Part model, mm, in its own coordinate system. A direction names the side the tool comes from. Round coordinates to 2 decimals unless told otherwise and drop trailing zeros. Loops run counter-clockwise (first coordinate to the right, second up) from the corner with the lowest first, then second, coordinate; pieces in that order, holes last.
Autodesk Inventor part; units mm, degrees
ref_plane "YZ Plane" through (0, 0, 0) normal (1, 0, 0) x (0, 1, 0)
ref_plane "XZ Plane" through (0, 0, 0) normal (0, 1, 0) x (-1, 0, 0)
ref_plane "XY Plane" through (0, 0, 0) normal (0, 0, 1) x (1, 0, 0)
sketch "Sketch3" plane through (0, 0, 0) normal (0, 1, 0) x (-1, 0, 0)
  line L0 (0, 0) -> (-55, 0)
  line L1 (-55, 0) -> (-55, -35.25)
  line L2 (-55, -35.25) -> (0, -35.25)
  line L3 (0, -35.25) -> (0, 0)
  line L4 (1.5, 1.5) -> (-56.5, 1.5)
  line L5 (-56.5, 1.5) -> (-56.5, -36.75)
  line L6 (-56.5, -36.75) -> (1.5, -36.75)
  line L7 (1.5, -36.75) -> (1.5, 1.5)
  dimension "d0" = 35.25
  dimension "d1" = 55
  dimension "d4" = 38.25
  dimension "d5" = 58
  dimension "d6" = 1.5
  dimension "d7" = 1.5
extrude "Extrusion1" add sketch "Sketch3" against normal blind 1.5 contours L3 L2 L1 L0 | L7 L6 L5 L4
sketch "Sketch5" plane through (0, 0, 0) normal (0, 1, 0) x (-1, 0, 0)
  line L0 (-55, 0) -> (-55, -35.25)
  line L1 (-55, -35.25) -> (0, -35.25)
  line L2 (0, -35.25) -> (0, 0)
  line L3 (-56.5, 1.5) -> (-56.5, -36.75)
  line L4 (-56.5, -36.75) -> (1.5, -36.75)
  line L5 (1.5, -36.75) -> (1.5, 1.5)
  line L6 (0, 0) -> (0, 1.5)
  line L7 (1.5, 1.5) -> (0, 1.5)
  line L8 (-55, 0) -> (-55, 1.5)
  line L9 (-55, 1.5) -> (-56.5, 1.5)
  dimension "d9" = 55
  dimension "d11" = 58
  dimension "d12" = 1.5
extrude "Extrusion2" add sketch "Sketch5" along normal blind 28
sketch "Sketch6" plane through (0, 28, 0) normal (0, 1, 0) x (1, 0, 0)
  line L0 (-1.5, -1.5) -> (56.5, -1.5)
  line L1 (56.5, -1.5) -> (56.5, 36.75)
  line L2 (56.5, 36.75) -> (-1.5, 36.75)
  line L3 (-1.5, 36.75) -> (-1.5, -1.5)
  point P0 (0, 0)
extrude "Extrusion3" add sketch "Sketch6" along normal blind 1.5
sketch "Sketch7" plane through (0, 0, 1.5) normal (1, 0, 0) x (0, 0, -1)
  line L0 (8.375, 4.5) -> (23.375, 4.5)
  line L1 (23.375, 4.5) -> (23.375, 5.5)
  line L2 (23.375, 5.5) -> (8.375, 5.5)
  line L3 (8.375, 5.5) -> (8.375, 4.5)
  line L4 (36.75, 0) -> (36.75, 28)
  line L5 (0, 0) -> (0, 28)
  line L6 (36.75, 0) -> (0, 0)
  point P0 (1.5, 0)
  dimension "d20" = 15
  dimension "d21" = 1
  dimension "d22" = 13.375
  dimension "d23" = 8.375
  dimension "d40" = 4.5
ref_plane "Work Plane1" through (27.5, 0, 1.5) normal (1, 0, 0) x (0, 0, -1)
extrude "Extrusion4" add sketch "Sketch7" along normal blind 2
mirror "Mirror1" about plane through (27.5, 0, 1.5) normal (1, 0, 0) of "Extrusion4"
sketch "Sketch8" plane through (-1.5, -1.5, 1.5) normal (0, 0, 1) x (1, 0, 0)
  line L0 (0.75, 30.25) -> (57.25, 30.25)
  line L1 (57.25, 30.25) -> (57.25, 13.25)
  line L2 (0.75, 13.25) -> (0.75, 30.25)
  line L3 (0, 31) -> (58, 31)
  line L4 (0.75, 13.25) -> (0, 13.25)
  line L5 (57.25, 13.25) -> (58, 13.25)
  line L6 (0, 31) -> (0, 13.25)
  line L7 (0, 31) -> (0, 0)
  line L8 (58, 31) -> (58, 13.25)
  line L9 (58, 0) -> (58, 31)
  point P0 (1.5, 1.5)
  dimension "d27" = 0.75
  dimension "d29" = 56.5
  dimension "d31" = 17
  dimension "d65" = 0.75
  dimension "d84" = 17
extrude "Extrusion5" add sketch "Sketch8" along normal blind 3
sketch "Sketch9" plane through (-1.5, -1.5, 1.5) normal (0, 0, 1) x (1, 0, 0)
  line L0 (0.75, 0.75) -> (57.25, 0.75)
  line L1 (57.25, 0.75) -> (57.25, 17.5)
  line L2 (0.75, 17.5) -> (0.75, 0.75)
  line L3 (1.5, 1.5) -> (56.5, 1.5)
  line L4 (57.25, 17.5) -> (56.5, 17.5)
  line L5 (56.5, 1.5) -> (56.5, 29.5)
  line L6 (56.5, 1.5) -> (56.5, 17.5)
  line L7 (56.5, 1.5) -> (1.5, 1.5)
  line L8 (0.75, 17.5) -> (1.5, 17.5)
  line L9 (1.5, 1.5) -> (1.5, 29.5)
  line L10 (1.5, 17.5) -> (1.5, 1.5)
  line L11 (1.5, 29.5) -> (56.5, 29.5)
  dimension "d34" = 0.75
  dimension "d36" = 56.5
  dimension "d69" = 16.75
  dimension "d70" = 16.75
  dimension "d97" = 28.75
extrude "Extrusion6" add sketch "Sketch9" along normal blind 3 contours L2 L8 L9 L3 L5 L4 L1 L0
sketch "Sketch10" plane through (0, 0, -35.25) normal (0, 0, 1) x (1, 0, 0)
  line L0 (55, 0) -> (0, 0)
  line L1 (20.5, 0) -> (34.5, 0)
  line L2 (34.5, 0) -> (34.5, 3.3)
  line L3 (34.5, 3.3) -> (20.5, 3.3)
  line L4 (20.5, 3.3) -> (20.5, 0)
  line L5 (0, 0) -> (0, 28)
  dimension "d41" = 14
  dimension "d42" = 20.5
  dimension "d43" = 3.3
extrude "Extrusion7" add sketch "Sketch10" along normal blind 5
fillet "Fillet1" radius 1 8 edges at (56.5, 29.5, -16.125) (56.5, -1.5, -17.625) (56.5, 14, -36.75) (27.5, 29.5, -36.75) (27.5, -1.5, -36.75) (-1.5, 14, -36.75) (-1.5, 29.5, -16.125) (-1.5, -1.5, -17.625)
sketch "Sketch11" plane through (0, 28, -35.25) normal (0, 0, 1) x (1, 0, 0)
  circle A0 centre (27.5, -17.2) radius 4.95
  line L0 (20.5, -24.7) -> (34.5, -24.7)
  line L1 (0, -28) -> (0, 0)
  dimension "d47" = 9.9
  dimension "d48" = 7.5
  dimension "d49" = 27.5
extrude "Extrusion8" cut sketch "Sketch11" against normal blind 5
fillet "Fillet2" radius 1 1 edges at (-0.75, -0.75, 3)
fillet "Fillet3" radius 1 1 edges at (55.75, -0.75, 3)
sketch "Sketch15" plane through (56.5, 11.75, 4.5) normal (1, 0, 0) x (0, 0, -1)
  line L0 (0, 0) -> (5, 0)
  line L1 (5, 0) -> (5, 12.75)
  line L2 (5, 12.75) -> (0, 12.75)
  line L3 (0, 12.75) -> (0, 0)
  line L4 (5, 0) -> (3, 0)
  line L5 (3, 0) -> (3, -7.25)
  line L6 (3, -7.25) -> (5, -7.25)
  line L7 (5, -7.25) -> (5, 0)
  point P0 (4.5, -11.75)
  point P1 (0, 4.25)
  point P2 (0, 17.75)
  dimension "d78" = 5
  dimension "d79" = 12.75
  dimension "d80" = 2
  dimension "d81" = 7.25
  dimension "d98" = 11.5
  dimension "d99" = 20
  dimension "d100" = 12.75
  dimension "d101" = 5
extrude "Extrusion10" add sketch "Sketch15" along normal blind 5
mirror "Mirror3" about plane through (27.5, 0, 1.5) normal (1, 0, 0) of "Extrusion10"
fillet "Fillet7" radius 1 2 edges at (61.5, 24.5, 2) (61.5, 4.5, 0.5)
fillet "Fillet8" radius 1 2 edges at (-6.5, 24.5, 2) (-6.5, 4.5, 0.5)
sketch "Sketch16" plane through (-1.5, -1.5, 4.5) normal (0, 0, 1) x (1, 0, 0)
  circle A0 centre (60.5, 22.5) radius 1.5
  line L0 (63, 25) -> (63, 13.25)
  line L1 (58, 26) -> (62, 26)
  point P0 (1.5, 1.5)
  dimension "d87" = 3
  dimension "d88" = 2.5
  dimension "d89" = 3.5
extrude "Extrusion11" cut sketch "Sketch16" against normal blind 5
sketch "Sketch17" plane through (-0.5, -1.5, 1.5) normal (0, 0, 1) x (1, 0, 0)
  circle A0 centre (59.5, 9.5) radius 1.5
  line L0 (57, 6) -> (61, 6)
  line L1 (62, 7) -> (62, 25)
  point P0 (0.5, 1.5)
  dimension "d92" = 3
  dimension "d93" = 3.5
  dimension "d94" = 2.5
extrude "Extrusion12" cut sketch "Sketch17" against normal blind 2
mirror "Mirror4" about plane through (27.5, 0, 1.5) normal (1, 0, 0) of "Extrusion11", "Extrusion12"
equation "\"d7\" = d6"
equation "\"d31\" = d66"
equation "\"d70\" = d69"
properties part number "sensor1_2t"
1) Drop flat-ended pins along their axis: pin 1 Ø1 at (y, z) = (7, -30) entering from -X; pin 2 Ø3 at (x, z) = (57.5, 2.5) entering from +Y; pin 3 Ø0.9 at (x, z) = (15.5, 3) entering from -Y; pin 4 Ø6 at (x, y) = (27.5, 10.8) entering from +Z. Give the stop position or say it passes through.
Values:
pin 1: stops at x = -1.5
pin 2: stops at y = 29.37
pin 3: stops at y = -0.75
pin 4: passes through
2) Tool access for faces 1 (the face through (-0.75, 6, 3)), 2 (the face through (-4, 15, -0.5)), 3 (the face through (1, 5.5, -14)): list every direction of +Z, -Z, +X, -X, +Y, -Y with a clear straight run to the whole face (end or side of a thin tool).
Values:
face 1: +Z, -X, -Y
face 2: -Z, -X, +Y, -Y
face 3: +Z
3) Slice it at A-A, the plane x = 27.5. Give the cut face in (y, z).
Values:
outline: (-1.5, -35.75) arc R1 ccw to (-0.5, -36.75) - (5.85, -36.75) - (5.85, -35.25) - (3.3, -35.25) - (3.3, -30.25) - (0, -30.25) - (0, 4.5) - (-0.75, 4.5) - (-0.75, 1.5) - (-1.5, 1.5) - close; (15.75, -36.75) - (28.5, -36.75) arc R1 ccw to (29.5, -35.75) - (29.5, 4.5) - (28.75, 4.5) - (28.75, 1.5) - (28, 1.5) - (28, -35.25) - (15.75, -35.25) - close
4) Wall check: line 1 along Y through (x, z) = (59, 0); line 2 along Y through (x, z) = (26, -22.5); line 3 along X through (y, z) = (11, -11). Give the ranges that are in metal, low to high.
Values:
line 1: y = 4.5 to 6.5, 9.5 to 19.5, 22.5 to 24.5
line 2: y = -1.5 to 0, 28 to 29.5
line 3: x = -1.5 to 0, 55 to 56.5
5) Slice it at B-B, the plane y = 21. Give the cut face in (x, z), then the cut area to 3 significant figures.
Values:
outline: (-6.5, -0.5) - (-5.5, -0.5) - (-5.5, 4.5) - (-6.5, 4.5) - close; (-2.5, -0.5) - (-1.5, -0.5) - (-1.5, -35.75) arc R1 ccw to (-0.5, -36.75) - (55.5, -36.75) arc R1 ccw to (56.5, -35.75) - (56.5, -0.5) - (57.5, -0.5) - (57.5, 4.5) - (55.75, 4.5) - (55.75, 1.5) - (55, 1.5) - (55, -35.25) - (0, -35.25) - (0, 1.5) - (-0.75, 1.5) - (-0.75, 4.5) - (-2.5, 4.5) - close; (60.5, -0.5) - (61.5, -0.5) - (61.5, 4.5) - (60.5, 4.5) - close
area: 221 mm2
6) Slice it at D-D, the plane z = -6. Give the cut face in (x, y), then the cut area to 3 significant figures.
Values:
outline: (-1.5, -0.5) arc R1 ccw to (-0.5, -1.5) - (55.5, -1.5) arc R1 ccw to (56.5, -0.5) - (56.5, 28.5) arc R1 ccw to (55.5, 29.5) - (-0.5, 29.5) arc R1 ccw to (-1.5, 28.5) - close; hole (0, 0) - (55, 0) - (55, 28) - (0, 28) - close
area: 257 mm2
7) Mould opens along X. For faces 4 (the face through (56.5, 14, -15)), 5 (the face through (27, 2, -30.25)), 6 (the face through (-6.5, 17, 2)), 7 (the face through (28, -1.5, -17)) say: released by +X, released by -X, zero draft, split by the parting line, or undercut.
Values:
face 4: released by +X
face 5: undercut
face 6: released by -X
face 7: zero draft
8) Slice it at C-C, the plane x = -4. Give the cut face in (y, z), then the cut area to 4 significant figures.
Values:
outline: (4.5, -0.5) - (6.5, -0.5) - (6.5, 1.5) - (4.5, 1.5) - close; (9.5, -0.5) - (19.5, -0.5) - (19.5, 4.5) - (11.75, 4.5) - (11.75, 1.5) - (9.5, 1.5) - close; (22.5, -0.5) - (24.5, -0.5) - (24.5, 4.5) - (22.5, 4.5) - close
area: 57.25 mm2
